Geometry: final body of the model. Coordinates: model frame, mm. Face numbers are marked on the shaded views. A direction names the side the tool comes from. Give positions to 0.01 mm unless a question says otherwise; leave off trailing zeros. Write each loop counter-clockwise with the first axis right and the second up, starting at its lowest first coordinate (ties: lowest second). Pieces come first, ordered by that corner, then holes.
Q1. Section C-C (x = 11.25). Return the cut outline in (y, z), plus the area to 3 significant figures.
Q2. Reachability of the marked faces 1 and 2 from +Z, -Z, +X, -X, +Y, -Y: full face, straight path, thin tool, end or side. Return the list, or none.
Q3. Pin query (flat end, axial travel): pin 1 Ø2 at (x, y) = (16.5, 45) entering from -Z; pin 2 Ø10 at (x, z) = (7, 17.5) entering from -Y; pin 3 Ø2.5 at (x, z) = (12, -4) entering from +Y. Return the tip coordinate at first contact, or that it passes through.
Q4. Section B-B (z = -4.5). Return the cut outline in (x, y), plus the area to 3 significant figures.
Q5. Section A-A (x = 15). Return the cut outline in (y, z).
Q6. Line query: line 1 (Y direction, x = 13.75, z = -3); line 2 (Y direction, x = 15.75, z = 5.5); line 3 (Z direction, x = 7, y = 32). Output: solid intervals per line, ascending.
Q7. Section D-D (y = 30). Return the cut outline in (x, z), plus the area to 3 significant figures.
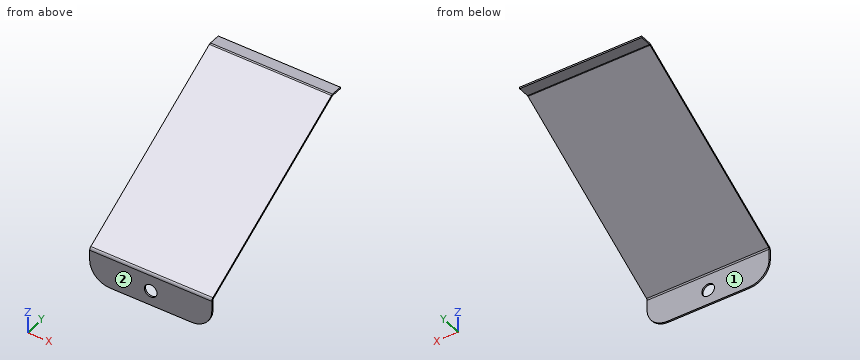
from build123d import *

# Parameters (mm, degrees)
BOSS_EXTRUDE1_DEPTH          = 30
EDGE_FLANGE1_DEPTH           = 30
EDGE_FLANGE1_2_DEPTH         = 30
EDGE_FLANGE2_STRIP_CUT_DEPTH = 30
EDGE_FLANGE2_DEPTH           = 30
SKETCH12_R                   = 1.55
CUT_EXTRUDE1_DEPTH           = 61.278165958
FILLET1_R                    = 5


# Read off the part's stored shape, not the designer's step: Edge-Flange1
# Sheet-metal steps are written as plain solids
with BuildPart() as part:
    # Sketch1 → Boss-Extrude1 (new body)
    with BuildSketch(Plane(origin=(0, 0, 0), x_dir=(0, 0, -1), z_dir=(1, 0, 0))):
        Polygon((-24.826638925, 43.401), (-25.173049087, 43.201), (-0.173205081, -0.1), (0.173205081, 0.1), align=None)
    extrude(amount=BOSS_EXTRUDE1_DEPTH)

    # Edge-Flange1 outline → Edge-Flange1 (cut)
    with BuildSketch(Plane.YZ):
        with BuildLine():
            Line((-0.1, 0.173205081), (0.1, -0.173205081))
            ThreePointArc((0.1, -0.173205081), (0.207179677, 0.226794919), (0.5, 0.519615242))
            Line((0.5, 0.519615242), (-0.1, 0.173205081))
        make_face()
    extrude(amount=EDGE_FLANGE1_DEPTH, mode=Mode.SUBTRACT)

    # Edge-Flange1 2 outline → Edge-Flange1 2 (add)
    with BuildSketch(Plane.YZ):
        with BuildLine():
            Line((0.7, 0.173205081), (0.1, -0.173205081))
            Line((0.1, -0.173205081), (0.1, -7.711324865))
            Line((0.1, -7.711324865), (0.5, -7.711324865))
            Line((0.5, -7.711324865), (0.5, -0.173205081))
            ThreePointArc((0.5, -0.173205081), (0.553589838, 0.026794919), (0.7, 0.173205081))
        make_face()
    extrude(amount=EDGE_FLANGE1_2_DEPTH)

    # Edge-Flange2 strip (across the edge) → Edge-Flange2 strip cut (cut)
    with BuildSketch(Plane(origin=(0, 43.401, 24.826638925), x_dir=(0, 0, -1), z_dir=(1, 0, 0))):
        Polygon((-1.492820323, 1.785640646), (-0.292820323, -0.292820323), (0.053589838, -0.092820323), (-1.146410162, 1.985640646), align=None)
    extrude(amount=EDGE_FLANGE2_STRIP_CUT_DEPTH, mode=Mode.SUBTRACT)

    # Edge-Flange2 section (across the edge) → Edge-Flange2 (add)
    with BuildSketch(Plane(origin=(0, 43.401, 24.826638925), x_dir=(0, 0, -1), z_dir=(1, 0, 0))):
        with BuildLine():
            Line((-0.4, 0.107179677), (-0.4, 2.892820323))
            Line((-0.4, 2.892820323), (0, 2.892820323))
            Line((0, 2.892820323), (0, 0.107179677))
            ThreePointArc((0, 0.107179677), (0.013629669, 0.003652059), (0.053589838, -0.092820323))
            Line((0.053589838, -0.092820323), (-0.292820323, -0.292820323))
            ThreePointArc((-0.292820323, -0.292820323), (-0.372740661, -0.099875559), (-0.4, 0.107179677))
        make_face()
    extrude(amount=EDGE_FLANGE2_DEPTH)

    # Sketch12 → Cut-Extrude1 (cut, through all)
    with BuildSketch(Plane(origin=(0, 0.5, 0), x_dir=(1, 0, 0), z_dir=(0, 1, 0))):
        with Locations(Location((15, 4.057735027, 0), (0, 0, 270))):
            Circle(SKETCH12_R)
    extrude(amount=-CUT_EXTRUDE1_DEPTH, mode=Mode.SUBTRACT)

    # Fillet1
    fillet1_edges = [part.edges().sort_by_distance(p)[0] for p in [
        (30, 0.3, -7.711324865),
        (0, 0.3, -7.711324865),
    ]]
    fillet(fillet1_edges, radius=FILLET1_R)


solid = part.part
Computed:
1. outline: (0.1, -7.71) - (0.5, -7.71) - (0.5, -0.17) arc R0.4 cw to (0.7, 0.17) - (43.31, 24.77) arc R0.4 cw to (43.51, 24.83) - (46.29, 24.83) - (46.29, 25.23) - (43.51, 25.23) arc R0.8 ccw to (43.11, 25.12) - (0.5, 0.52) arc R0.8 ccw to (0.1, -0.17) - close
1. area: 24.2 mm2
2. face 1: -Z, +X, -X, +Y
2. face 2: +Z, -Z, +X, -X, -Y
3. pin 1: stops at z = 24.83
3. pin 2: stops at y = 21.25
3. pin 3: stops at y = 0.5
4. outline: (0.33, 0.1) - (13.51, 0.1) - (13.51, 0.5) - (0.33, 0.5) - close; (16.49, 0.1) - (29.67, 0.1) - (29.67, 0.5) - (16.49, 0.5) - close
4. area: 10.5 mm2
5. outline: (0.1, -7.71) - (0.5, -7.71) - (0.5, -5.61) - (0.1, -5.61) - close; (0.1, -2.51) - (0.5, -2.51) - (0.5, -0.17) arc R0.4 cw to (0.7, 0.17) - (43.31, 24.77) arc R0.4 cw to (43.51, 24.83) - (46.29, 24.83) - (46.29, 25.23) - (43.51, 25.23) arc R0.8 ccw to (43.11, 25.12) - (0.5, 0.52) arc R0.8 ccw to (0.1, -0.17) - close
6. line 1: y = 0.1 to 0.5
6. line 2: y = 9.13 to 9.93
6. line 3: z = 18.24 to 18.71
7. outline: (0, 17.09) - (30, 17.09) - (30, 17.55) - (0, 17.55) - close
7. area: 13.9 mm2
